Here's how the part is built. I have some questions about the finished solid (model axes, mm). A direction names the side the tool comes from. Give positions to 0.01 mm unless a question says otherwise; leave off trailing zeros. Write each loop counter-clockwise with the first axis right and the second up, starting at its lowest first coordinate (ties: lowest second). Pieces come first, ordered by that corner, then holes. Notation, with made-up numbers: (4, 45) -> (54, 45) arc R25 cw to (54, 77) -> close; hole circle Ø3 at (-19.5, -4). An arc over 180 degrees is marked (long way). Use CSV: the item, a comma, the result in double quotes. Start each with the question number.
(1) Suppose I cut it at A-A on x = -273.5. List the corners of the cut face in (y, z) for me.
(2) Suppose I cut it at B-B on y = 140. List the corners of the cut face in (x, z) for me.
(3) I need wall thicknesses on L1, parallel to Y at x = -312.5, z = 4.35; L2, parallel to X at y = 85, z = 1.3; L3, parallel to Y at x = -243, z = 3.3. Which ranges of each line are inside material? Lowest first, please. Write a range as [from, to].
(4) If we mould it in two halves opening along X, with no side actions, what happens to faces 3 (the flat face through (-412.793, 118, 3)), 4 (the flat face through (-297, 14.859, 3)), 5 (the flat face through (-299, 234.859, 3))? For each: pulls with the +X half, pulls with the -X half, needs draft (parallel to the pull), parting line crosses it, or undercut.
(5) Which directions (+Z, -Z, +X, -X, +Y, -Y) give clear straight access to the entire face, cutting with the end or side of a thin tool? Please do faces 1 (the flat face through (-299, 4.859, 3)), 2 (the flat face through (-372.47, 193.674, 2.958)).
(6) Suppose I cut it at C-C on z = 4.55. List the corners of the cut face in (x, y) for me.
from build123d import *

# Parameters (mm, degrees)
F0_W     = 230
F0_H     = 230
F0_R     = 1.5
F1_DEPTH = 6


with BuildPart() as f1:
    # F0 (on Top) → F1 (new body)
    with BuildSketch(Plane.XY):
        with Locations((-297.792881, 119.858589)):
            Rectangle(F0_W, F0_H)
        with Locations((-397.792881, 219.858589)):
            Circle(F0_R, mode=Mode.SUBTRACT)
        Polygon((-402.792881, 163.351013), (-341.285305, 224.858589), (-254.300457, 224.858589), (-192.792881, 163.351013), (-192.792881, 76.366165), (-254.300457, 14.858589), (-341.285305, 14.858589), (-402.792881, 76.366165), align=None, mode=Mode.SUBTRACT)
    extrude(amount=F1_DEPTH)


solid = f1.part
Geometry says:
1,outline,"(4.86, 0) -> (14.86, 0) -> (14.86, 6) -> (4.86, 6) -> close; (224.86, 0) -> (234.86, 0) -> (234.86, 6) -> (224.86, 6) -> close"
2,outline,"(-412.79, 0) -> (-402.79, 0) -> (-402.79, 6) -> (-412.79, 6) -> close; (-192.79, 0) -> (-182.79, 0) -> (-182.79, 6) -> (-192.79, 6) -> close"
3,L1,"[4.86, 14.86], [224.86, 234.86]"
3,L2,"[-412.79, -402.79], [-192.79, -182.79]"
3,L3,"[4.86, 26.16], [213.56, 234.86]"
4,face 3,"pulls with the -X half"
4,face 4,"undercut"
4,face 5,"needs draft"
5,face 1,"+Z, -Z, +X, -X, -Y"
5,face 2,"+Z, -Z"
6,outline,"(-412.79, 4.86) -> (-182.79, 4.86) -> (-182.79, 234.86) -> (-412.79, 234.86) -> close; hole (-402.79, 76.37) -> (-341.29, 14.86) -> (-254.3, 14.86) -> (-192.79, 76.37) -> (-192.79, 163.35) -> (-254.3, 224.86) -> (-341.29, 224.86) -> (-402.79, 163.35) -> close; hole circle Ø3 at (-397.79, 219.86)"
